from build123d import *

# Parameters (mm, degrees)
F0_W     = 60
F0_H     = 60
F1_DEPTH = 10
F2_R     = 10
F4_D     = 10
F5_R     = 16
F6_DEPTH = 20
F8_D     = 14


with BuildPart() as f1:
    # F0 (on Front) → F1 (new body)
    with BuildSketch(Plane.XZ):
        Rectangle(F0_W, F0_H)
    extrude(amount=F1_DEPTH)

    # F2
    f2_edges = [f1.edges().sort_by_distance(p)[0] for p in [
        (-30, -5, 30),
        (-30, -5, -30),
        (30, -5, 30),
        (30, -5, -30),
    ]]
    fillet(f2_edges, radius=F2_R)

    # F4 (through all)
    with Locations(Plane.XZ.offset(10)):
        with Locations((-20, 20), (20, 20), (20, -20), (-20, -20)):
            Hole(F4_D / 2)

    # F5 (on face) → F6 (join)
    with BuildSketch(Plane.XZ.offset(10)):
        Circle(F5_R)
    extrude(amount=F6_DEPTH)

    # F8 (through all)
    with Locations(Plane.XZ.offset(30)):
        with Locations((0, 0)):
            Hole(F8_D / 2)


solid = f1.part
Design review of the part built by this model. Coordinates are the model's own, in mm. A direction names the side the tool comes from. Round coordinates to 2 decimals unless told otherwise and drop trailing zeros. Write each loop counter-clockwise with the first axis right and the second up, starting at its lowest first coordinate (ties: lowest second). Pieces come first, ordered by that corner, then holes.
Item 1: Wall thickness on L1, parallel to Z at x = -20, y = -7.5; L2, parallel to X at y = -17.5, z = -0.5; L3, parallel to X at y = -1.5, z = -21.5: over which ranges is each line inside the solid? List them lowest first.
Item 2: Consider section C-C on x = -19. Give the boundary of the cut face in (y, z), and give its area (3 significant figures).
Item 3: For faces 1 (the flat face through (13, -10, -13)), 2 (the flat face through (-30, -5, 0)), list the 3-axis set-ups (+Z, -Z, +X, -X, +Y, -Y) from which the entire face can be reached by the end or side of a thin tool; tool diameter is ignored.
Item 4: Consider section A-A on z = 0. Give the boundary of the cut face in (x, y).
Item 5: Consider section D-D on y = -27.5. Give the boundary of the cut face in (x, z).
Item 6: For pin 1 Ø6 at (x, z) = (20, 20) entering from +Y; pin 2 Ø5 at (x, y) = (-8.5, -15) entering from -Z; pin 3 Ø2 at (x, z) = (19.5, -14.5) entering from -Y, all flat-tipped, find the tip position at first contact; note any pin that passes through.
Item 7: Consider section B-B on x = 2. Give the boundary of the cut face in (y, z), and give its area (3 significant figures).
Item 8: Draft analysis for pull direction X (two halves, no side actions). For faces 3 (the cylindrical face through (-18.92, -4.93, -24.88)), 4 (the flat face through (0, -5, 30)), 5 (the flat face through (30, -5, 0)), state which applies: released by +X, released by -X, zero draft, split by the parting line, or undercut.
Check values:
1. L1: z = -30 to -25, -15 to 15, 25 to 30
1. L2: x = -15.99 to -6.98, 6.98 to 15.99
1. L3: x = -29.89 to -24.77, -15.23 to 15.23, 24.77 to 29.89
2. outline: (-10, -30) - (0, -30) - (0, -24.9) - (-10, -24.9) - close; (-10, -15.1) - (0, -15.1) - (0, 15.1) - (-10, 15.1) - close; (-10, 24.9) - (0, 24.9) - (0, 30) - (-10, 30) - close
2. area: 404 mm2
3. face 1: -Y
3. face 2: +Z, -Z, -X, +Y, -Y
4. outline: (-30, -10) - (-16, -10) - (-16, -30) - (-7, -30) - (-7, 0) - (-30, 0) - close; (7, -30) - (16, -30) - (16, -10) - (30, -10) - (30, 0) - (7, 0) - close
5. outline: circle Ø32 at (0, 0); hole circle Ø14 at (0, 0)
6. pin 1: passes through
6. pin 2: stops at z = -14.83
6. pin 3: stops at y = -10
7. outline: (-30, -15.87) - (-10, -15.87) - (-10, -30) - (0, -30) - (0, -6.71) - (-30, -6.71) - close; (-30, 6.71) - (0, 6.71) - (0, 30) - (-10, 30) - (-10, 15.87) - (-30, 15.87) - close
7. area: 832 mm2
8. face 3: undercut
8. face 4: zero draft
8. face 5: released by +X
